Verification items for the finished model (mm, model axes). A direction names the side the tool comes from. Round coordinates to 2 decimals unless told otherwise and drop trailing zeros. Write each loop counter-clockwise with the first axis right and the second up, starting at its lowest first coordinate (ties: lowest second). Pieces come first, ordered by that corner, then holes. Notation, with made-up numbers: M 73,4 L 101,4 A18 ccw 101,23 Z; hole C -8.5,-0.5 d4. An arc over 180 degrees is marked long. Use a Markdown table: item, result. Add a question column.
from build123d import *

# Parameters (mm, degrees)
BOSS_EXTRUDE1_DEPTH = 160
CUT_EXTRUDE1_DEPTH  = 32
SKETCH3_R           = 7.5
CUT_EXTRUDE2_DEPTH  = 210
SKETCH5_R           = 1.5
CUT_EXTRUDE4_DEPTH  = 210
CUT_EXTRUDE6_DEPTH  = 20
SKETCH8_R           = 1.55
CUT_EXTRUDE7_DEPTH  = 10
SKETCH9_W           = 20
SKETCH9_H           = 12
BOSS_EXTRUDE3_DEPTH = 2
SKETCH10_W          = 3
SKETCH10_H          = 12
BOSS_EXTRUDE4_DEPTH = 25
SKETCH11_R          = 3.5
CUT_EXTRUDE8_DEPTH  = 1
SKETCH12_R          = 1.55
CUT_EXTRUDE9_DEPTH  = 3
SKETCH13_R          = 1.5
SKETCH13_R_2        = 1.55
CUT_EXTRUDE10_DEPTH = 10
SKETCH14_R          = 1.375
BOSS_EXTRUDE5_DEPTH = 5
SKETCH15_W          = 80
SKETCH15_H          = 42
CUT_EXTRUDE11_DEPTH = 5
FILLET1_R           = 7
SKETCH16_W          = 80
SKETCH16_H          = 42
CUT_EXTRUDE12_DEPTH = 5
FILLET2_R           = 7


with BuildPart() as part:
    # Sketch1 → Boss-Extrude1 (new body)
    with BuildSketch(Plane.XY):
        Polygon((-95.061728395, -14.551440329), (-95.061728395, 27.448559671), (54.938271605, 27.448559671), (54.938271605, -14.551440329), (49.938271605, -14.551440329), (49.938271605, 20.448559671), (-90.061728395, 20.448559671), (-90.061728395, -14.551440329), align=None)
    extrude(amount=BOSS_EXTRUDE1_DEPTH)

    # Sketch2 → Cut-Extrude1 (cut)
    with BuildSketch(Plane(origin=(0, 0, 0), x_dir=(-1, 0, 0), z_dir=(0, 0, -1))):
        with BuildLine():
            Line((-50.938271605, 15.448559671), (-50.938271605, -4.551440329))
            ThreePointArc((-50.938271605, -4.551440329), (-52.438271605, -6.051440329), (-53.938271605, -4.551440329))
            Line((-53.938271605, -4.551440329), (-53.938271605, 15.448559671))
            ThreePointArc((-53.938271605, 15.448559671), (-52.438271605, 16.948559671), (-50.938271605, 15.448559671))
        make_face()
        with BuildLine():
            Line((-4.938271605, 25.448559671), (45.061728395, 25.448559671))
            ThreePointArc((45.061728395, 25.448559671), (46.561728395, 23.948559671), (45.061728395, 22.448559671))
            Line((45.061728395, 22.448559671), (-4.938271605, 22.448559671))
            ThreePointArc((-4.938271605, 22.448559671), (-6.438271605, 23.948559671), (-4.938271605, 25.448559671))
        make_face()
        with BuildLine():
            Line((94.061728395, 15.448559671), (94.061728395, -4.551440329))
            ThreePointArc((94.061728395, -4.551440329), (92.561728395, -6.051440329), (91.061728395, -4.551440329))
            Line((91.061728395, -4.551440329), (91.061728395, 15.448559671))
            ThreePointArc((91.061728395, 15.448559671), (92.561728395, 16.948559671), (94.061728395, 15.448559671))
        make_face()
    extrude(amount=-CUT_EXTRUDE1_DEPTH, mode=Mode.SUBTRACT)

    # Sketch3 → Cut-Extrude2 (cut)
    with BuildSketch(Plane.ZY.offset(95.061728395)):
        with Locations((120, 7.448559671)):
            Circle(SKETCH3_R)
    extrude(amount=-CUT_EXTRUDE2_DEPTH, mode=Mode.SUBTRACT)

    # Sketch5 → Cut-Extrude4 (cut)
    with BuildSketch(Plane(origin=(0, 27.448559671, 0), x_dir=(1, 0, 0), z_dir=(0, 1, 0))):
        with Locations(Location((-80.061728395, -26.5, 0), (0, 0, 180))):
            Circle(SKETCH5_R)
        with Locations(Location((39.938271605, -26.5, 0), (0, 0, 180))):
            Circle(SKETCH5_R)
        with Locations(Location((-80.061728395, -86.5, 0), (0, 0, 180))):
            Circle(SKETCH5_R)
        with Locations(Location((39.938271605, -86.5, 0), (0, 0, 180))):
            Circle(SKETCH5_R)
    extrude(amount=-CUT_EXTRUDE4_DEPTH, mode=Mode.SUBTRACT)

    # Sketch7 → Cut-Extrude6 (cut)
    with BuildSketch(Plane(origin=(0, 27.448559671, 0), x_dir=(1, 0, 0), z_dir=(0, 1, 0))):
        with BuildLine():
            Line((-40.061728395, -102), (-0.061728395, -102))
            ThreePointArc((-0.061728395, -102), (3.938271605, -106), (-0.061728395, -110))
            Line((-0.061728395, -110), (-40.061728395, -110))
            ThreePointArc((-40.061728395, -110), (-44.061728395, -106), (-40.061728395, -102))
        make_face()
    extrude(amount=-CUT_EXTRUDE6_DEPTH, mode=Mode.SUBTRACT)

    # Sketch8 → Cut-Extrude7 (cut)
    with BuildSketch(Plane(origin=(0, 27.448559671, 0), x_dir=(1, 0, 0), z_dir=(0, 1, 0))):
        with Locations(Location((-75.061728395, -20, 0), (0, 0, 180))):
            Circle(SKETCH8_R)
        with Locations(Location((34.938271605, -20, 0), (0, 0, 180))):
            Circle(SKETCH8_R)
    extrude(amount=-CUT_EXTRUDE7_DEPTH, mode=Mode.SUBTRACT)

    # Sketch9 → Boss-Extrude3 (add)
    with BuildSketch(Plane.XZ.offset(-20.448559671)):
        with Locations((39.938271605, 100)):
            Rectangle(SKETCH9_W, SKETCH9_H)
    boss_extrude3 = extrude(amount=BOSS_EXTRUDE3_DEPTH)

    # Sketch10 → Boss-Extrude4 (add)
    with BuildSketch(Plane.XZ.offset(-18.448559671)):
        with Locations((31.438271605, 100)):
            Rectangle(SKETCH10_W, SKETCH10_H)
    boss_extrude4 = extrude(amount=BOSS_EXTRUDE4_DEPTH)

    # Sketch11 → Cut-Extrude8 (cut)
    with BuildSketch(Plane.ZY.offset(-29.938271605)):
        with Locations(Location((100, 15.948559671, 0), (0, 0, 270))):
            Circle(SKETCH11_R)
        with Locations(Location((100, -2.051440329, 0), (0, 0, 270))):
            Circle(SKETCH11_R)
    cut_extrude8 = extrude(amount=-CUT_EXTRUDE8_DEPTH, mode=Mode.SUBTRACT)

    # Sketch12 → Cut-Extrude9 (cut)
    with BuildSketch(Plane.ZY.offset(-30.938271605)):
        with Locations(Location((100, 15.948559671, 0), (0, 0, 270))):
            Circle(SKETCH12_R)
        with Locations(Location((100, -2.051440329, 0), (0, 0, 270))):
            Circle(SKETCH12_R)
    cut_extrude9 = extrude(amount=-CUT_EXTRUDE9_DEPTH, mode=Mode.SUBTRACT)

    # Mirror1: Boss-Extrude3, Boss-Extrude4, Cut-Extrude8, Cut-Extrude9 across plane
    add(boss_extrude3.mirror(Plane.ZY.offset(20.061728395)))
    add(boss_extrude4.mirror(Plane.ZY.offset(20.061728395)))
    add(cut_extrude8.mirror(Plane.ZY.offset(20.061728395)), mode=Mode.SUBTRACT)
    add(cut_extrude9.mirror(Plane.ZY.offset(20.061728395)), mode=Mode.SUBTRACT)

    # Sketch13 → Cut-Extrude10 (cut)
    with BuildSketch(Plane(origin=(0, 27.448559671, 0), x_dir=(1, 0, 0), z_dir=(0, 1, 0))):
        with Locations(Location((17.438271605, -37.265826534, 0), (0, 0, 180))):
            Circle(SKETCH13_R)
        with Locations(Location((-57.561728395, -37.265826534, 0), (0, 0, 180))):
            Circle(SKETCH13_R)
        with Locations(Location((-61.341728395, -67.223803809, 0), (0, 0, 180))):
            Circle(SKETCH13_R)
        with Locations(Location((21.218271605, -67.223803809, 0), (0, 0, 180))):
            Circle(SKETCH13_R_2)
    extrude(amount=-CUT_EXTRUDE10_DEPTH, mode=Mode.SUBTRACT)

    # Sketch14 → Boss-Extrude5 (add)
    # profile 1 of 2: a face of its own
    with BuildSketch(Plane.XZ.offset(-20.448559671)):
        with BuildLine():
            Line((5.139369782, 81.650400065), (5.139369782, 56.650400065))
            ThreePointArc((5.139369782, 56.650400065), (2.139369782, 53.650400065), (-0.860630218, 56.650400065))
            Line((-0.860630218, 56.650400065), (-0.860630218, 81.650400065))
            ThreePointArc((-0.860630218, 81.650400065), (2.139369782, 84.650400065), (5.139369782, 81.650400065))
        make_face()
        with Locations((2.139369782, 69.150400065)):
            Circle(SKETCH14_R, mode=Mode.SUBTRACT)
    # profile 2 of 2: a face of its own
    with BuildSketch(Plane.XZ.offset(-20.448559671)):
        with BuildLine():
            Line((-36.860630218, 81.650400065), (-36.860630218, 56.650400065))
            ThreePointArc((-36.860630218, 56.650400065), (-39.860630218, 53.650400065), (-42.860630218, 56.650400065))
            Line((-42.860630218, 56.650400065), (-42.860630218, 81.650400065))
            ThreePointArc((-42.860630218, 81.650400065), (-39.860630218, 84.650400065), (-36.860630218, 81.650400065))
        make_face()
        with Locations((-39.860630218, 69.150400065)):
            Circle(SKETCH14_R, mode=Mode.SUBTRACT)
    extrude(amount=BOSS_EXTRUDE5_DEPTH)

    # Sketch15 → Cut-Extrude11 (cut)
    with BuildSketch(Plane(origin=(54.938271605, 0, 0), x_dir=(0, 0, -1), z_dir=(1, 0, 0))):
        with Locations((-120, 6.448559671)):
            Rectangle(SKETCH15_W, SKETCH15_H)
    extrude(amount=-CUT_EXTRUDE11_DEPTH, mode=Mode.SUBTRACT)

    # Fillet1
    fillet1_edges = [part.edges().sort_by_distance(p)[0] for p in [
        (49.938271605, 27.448559671, 120),
    ]]
    fillet(fillet1_edges, radius=FILLET1_R - 0.0001)  # a hair under: the kernel refuses the full size

    # Sketch16 → Cut-Extrude12 (cut)
    with BuildSketch(Plane.ZY.offset(95.061728395)):
        with Locations((120, 6.448559671)):
            Rectangle(SKETCH16_W, SKETCH16_H)
    extrude(amount=-CUT_EXTRUDE12_DEPTH, mode=Mode.SUBTRACT)

    # Fillet2
    fillet2_edges = [part.edges().sort_by_distance(p)[0] for p in [
        (-90.061728395, 27.448559671, 120),
    ]]
    fillet(fillet2_edges, radius=FILLET2_R - 0.0001)  # a hair under: the kernel refuses the full size


solid = part.part
1. Access from +Z, -Z, +X, -X, +Y, -Y to the whole of each face (thin tool, end or side, straight path). Record for faces 4 (the flat face through (32.938, 6, 100)), 5 (the flat face through (-20, 24, 102)), 6 (the flat face through (32, 10, 106)).
2. Cross-section at A-A on x = -30. Enter the section's corners in (y, z), plus the area to 3 significant figures.
3. Scan lines: line 1 along X through (y, z) = (-7.5, 21); line 2 along Y through (x, z) = (-20, 16.5); line 3 along Y through (x, z) = (-21, 125.5). Record each from-to range of solid material in increasing order. Write a range as from..to.
4. Depth check by flat-ended pin: pin 1 Ø8 at (x, z) = (30, 103) entering from -Y; pin 2 Ø9.5 at (x, z) = (-81.5, 102.5) entering from -Y; pin 3 Ø2.5 at (x, z) = (39.94, 26.5) entering from -Y; pin 4 Ø12 at (y, z) = (8, 111.5) entering from +X. Enter the tip coordinate at first touch or a pass-through.
5. Cross-section at C-C on x = 27.5. Enter the section's corners in (y, z).
6. Cross-section at B-B on y = -11.5. Enter the section's corners in (x, z), plus the area to 3 significant figures.
7. Release check for a two-part mould opening along Y. For faces 1 (the flat face through (4, 15.449, 69)), 2 (the flat face through (-42.861, 18, 69)), 3 (the flat face through (-20, 22.449, 16)) record: +Y half, -Y half, draft (parallel to the pull), parting line (faces both ways), or undercut.
Answer:
| question | item | result |
|---|---|---|
| 1 | face 4 | +Z, -Z, +X, -Y |
| 1 | face 5 | +Y, -Y |
| 1 | face 6 | +Z, +X, -X, -Y |
| 2 | outline | M 20.45,0 L 22.45,0 L 22.45,32 L 25.45,32 L 25.45,0 L 27.45,0 L 27.45,102 L 20.45,102 Z; M 20.45,110 L 27.45,110 L 27.45,160 L 20.45,160 Z |
| 2 | area | 968 mm^2 |
| 3 | line 1 | x = -95.06..-90.06, 49.94..54.94 |
| 3 | line 2 | y = 20.45..22.45, 25.45..27.45 |
| 3 | line 3 | y = 20.45..27.45 |
| 4 | pin 1 | stops at y = -6.55 |
| 4 | pin 2 | stops at y = 18.45 |
| 4 | pin 3 | passes through |
| 4 | pin 4 | stops at x = 32.94 |
| 5 | outline | M 20.45,0 L 27.45,0 L 27.45,160 L 20.45,160 Z |
| 6 | outline | M -95.06,0 L -90.06,0 L -90.06,80 L -95.06,80 Z; M 49.94,0 L 54.94,0 L 54.94,80 L 49.94,80 Z |
| 6 | area | 800 mm^2 |
| 7 | face 1 | -Y half |
| 7 | face 2 | draft |
| 7 | face 3 | undercut |
